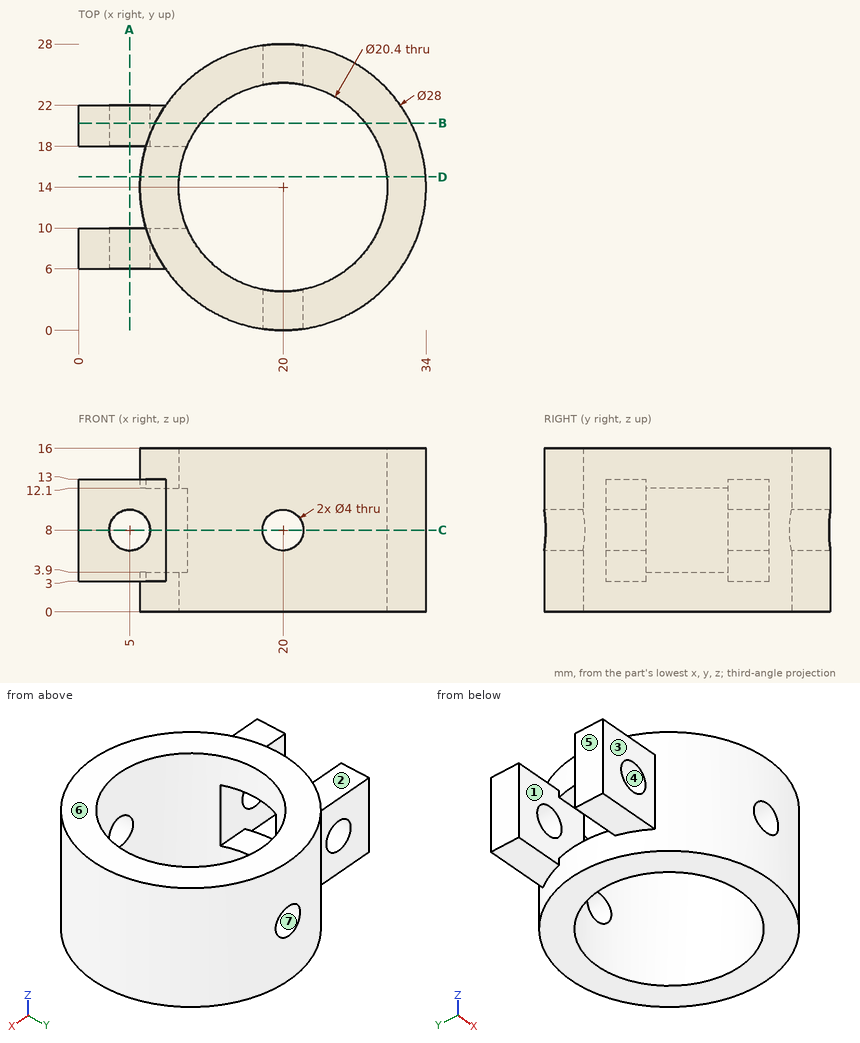
Print and shaded views of the part. All mm, measured from the part's lowest x, y and z. A direction names the side the tool comes from. Round coordinates to 2 decimals unless told otherwise and drop trailing zeros. Write each loop counter-clockwise with the first axis right and the second up, starting at its lowest first coordinate (ties: lowest second). Pieces come first, ordered by that corner, then holes. Notation, with made-up numbers: M 49.5,25 L 105.5,25 A25 cw 105.5,46 Z; hole C -22,24 d1. An arc over 180 degrees is marked long. One line per question, with ' | ' between items.
(1) Saw through at A-A on x = 5. Write the cut outline in (y, z), then the cut area to 3 significant figures.
Answer key:
outline: M 6,3 L 10,3 L 10,6 L 6,6 Z; M 6,10 L 10,10 L 10,13 L 6,13 Z; M 18,3 L 22,3 L 22,6 L 18,6 Z; M 18,10 L 22,10 L 22,13 L 18,13 Z | area: 48.0 mm^2
(2) Saw through at B-B on y = 20.25. Write the cut outline in (x, z), then the cut area to 3 significant figures.
Answer key:
outline: M 0,3 L 7.47,3 L 7.47,0 L 11.94,0 L 11.94,16 L 7.47,16 L 7.47,13 L 0,13 Z; M 28.06,0 L 32.53,0 L 32.53,16 L 28.06,16 Z; hole C 5,8 d4 | area: 205 mm^2
(3) 3-axis set-ups, long thin cutter, end or side, ignore diameter. For the marked faces 1, 2 and 3: which of +Z, -Z, +X, -X, +Y, -Y reach the whole face in a straight line?
Answer key:
face 1: -X | face 2: +Z, -X, +Y | face 3: +Z, -Z, -X, -Y
(4) Two-plate mould, pull along X, no slides. Class the marked faces 4, 5, 6 and 7: released by +X, released by -X, zero draft, split by the parting line, or undercut.
Answer key:
face 4: undercut | face 5: released by -X | face 6: zero draft | face 7: undercut
(5) Pin check, flat tips, straight feed: pin 1 (7 mm diameter, centred on x = 3, z = 8.5, fed in from +Y); pin 2 (8 mm diameter, centred on x = 15, z = 12.5, fed in from +Y); pin 3 (2 mm diameter, centred on x = 2.5, y = 20.5, fed in from -Z); pin 4 (8 mm diameter, centred on y = 17, z = 9, fed in from -X). Stop position of each tip, or through.
Answer key:
pin 1: stops at y = 22 | pin 2: stops at y = 27.96 | pin 3: stops at z = 3 | pin 4: stops at x = 0
(6) Probe line 1 along Z through (x, y) = (20, 25.95); line 2 along Z through (x, y) = (8, 13.25); line 3 along Y through (x, z) = (20, 4.75). List the from-to ranges inside material, lowest first.
Answer key:
line 1: z = 0 to 6, 10 to 16 | line 2: z = 0 to 3.9, 12.1 to 16 | line 3: y = 0 to 3.8, 24.2 to 28
(7) Saw through at C-C on z = 8. Write the cut outline in (x, y), then the cut area to 3 significant figures.
Answer key:
outline: M 0,6 L 3,6 L 3,10 L 0,10 Z; M 0,18 L 3,18 L 3,22 L 0,22 Z; M 7,6 L 8.51,6 A14 ccw 18,0.14 L 18,4 A10.2 cw 10.62,10 L 7,10 Z; M 7,18 L 10.62,18 A10.2 cw 18,24 L 18,27.86 A14 ccw 8.51,22 L 7,22 Z; M 22,0.14 A14 ccw 22,27.86 L 22,24 A10.2 cw 22,4 Z | area: 255 mm^2
(8) Saw through at D-D on y = 15. Write the cut outline in (x, z), then the cut area to 3 significant figures.
Answer key:
outline: M 6.04,0 L 9.85,0 L 9.85,3.9 L 6.04,3.9 Z; M 6.04,12.1 L 9.85,12.1 L 9.85,16 L 6.04,16 Z; M 30.15,0 L 33.96,0 L 33.96,16 L 30.15,16 Z | area: 90.8 mm^2
